Work out the finished part from the listing and answer in its coordinate system (mm). A direction names the side the tool comes from. Coordinates: 2 decimals unless noted, no trailing zeros. Order: outer loops, then holes, each group sorted by start corner. A loop starts at its lowest first (then second) coordinate and runs counter-clockwise, first axis right, second up. Notation, with made-up numbers: (46.5, 71) -> (58.5, 71) arc R26 ccw to (58.5, 99) -> close; hole circle Ø9 at (78.25, 2.5). An arc over 180 degrees is marked (long way). Answer as CSV lines item,"result". Start each with the question number.
Item 1: For a pull along Y with two mould halves and no side action, classify faces 4 (the face through (283, 139.7, 19)), 5 (the face through (343.184, 71.525, 19.317)), 6 (the face through (571.5, 70, 19)) as pulls with the +Y half, pulls with the -Y half, needs draft (parallel to the pull), parting line crosses it, or undercut.
Item 2: Straight lines are drawn through the part: L1, parallel to X at y = 72, z = 19; L2, parallel to Z at x = 527, y = 76; L3, parallel to Y at x = 366, z = 22. For each, find the intervals that lie inside material, in ascending order.
Item 3: Section D-D (y = 99.5) is taken. Write down the section's boundary in (x, z).
Item 4: Section B-B (z = 19.05) is taken. Write down the section's boundary in (x, y).
Item 5: Section C-C (x = 44.45) is taken. Write down the section's boundary in (y, z), then the cut area to 3 significant figures.
Item 6: Section A-A (y = 69.85) is taken. Count the separate pieces of the cut face and the enclosed holes in it, then the cut area to 3 significant figures.
Item 7: Which of the six approach directions +Z, -Z, +X, -X, +Y, -Y give full straight-line access (tool end or side, diameter ignored) to faces 1 (the face through (44, 50.8, 28)), 2 (the face through (526, 50.8, 28)), 3 (the face through (88.9, 114, 19))?
Item 8: Each of these flat-tipped pins is pushed along its axis until it touches: pin 1 Ø19 at (y, z) = (125, 27.5) entering from +X; pin 2 Ø19 at (x, z) = (54.5, 19.5) entering from +Y; pin 3 Ø2 at (y, z) = (122, 4) entering from -X; pin 4 Ø1.5 at (y, z) = (76, 14) entering from -X. Where does it stop, or does it pass through?
```python
from build123d import *

# Parameters (mm, degrees)
SKETCH2_W           = 571.5
SKETCH2_H           = 139.7
BOSS_EXTRUDE2_DEPTH = 38.1
SKETCH3_W           = 88.9
SKETCH3_H           = 50.8
CUT_EXTRUDE1_DEPTH  = 590.559114933
SKETCH4_R           = 38.1
CUT_EXTRUDE2_DEPTH  = 590.559114933
SKETCH5_R           = 4.7625
CUT_EXTRUDE3_DEPTH  = 580.626664328
SKETCH6_R           = 4.7625
CUT_EXTRUDE4_DEPTH  = 580.626664328


with BuildPart() as part:
    # Sketch2 → Boss-Extrude2 (new body)
    with BuildSketch(Plane.XY):
        with Locations((285.75, 69.85)):
            Rectangle(SKETCH2_W, SKETCH2_H)
    extrude(amount=BOSS_EXTRUDE2_DEPTH)

    # Sketch3 → Cut-Extrude1 (cut, through all)
    with BuildSketch(Plane.XY.offset(38.1)):
        with Locations((44.45, 114.3)):
            Rectangle(SKETCH3_W, SKETCH3_H)
        with Locations((527.05, 114.3)):
            Rectangle(SKETCH3_W, SKETCH3_H)
        with Locations((527.05, 25.4)):
            Rectangle(SKETCH3_W, SKETCH3_H)
        with Locations((44.45, 25.4)):
            Rectangle(SKETCH3_W, SKETCH3_H)
    extrude(amount=-CUT_EXTRUDE1_DEPTH, mode=Mode.SUBTRACT)

    # Sketch4 → Cut-Extrude2 (cut, through all)
    with BuildSketch(Plane.XY.offset(38.1)):
        with Locations((381.247583626, 69.85)):
            Circle(SKETCH4_R)
    extrude(amount=-CUT_EXTRUDE2_DEPTH, mode=Mode.SUBTRACT)

    # Sketch5 → Cut-Extrude3 (cut, through all)
    with BuildSketch(Plane(origin=(0, 50.8, 0), x_dir=(-1, 0, 0), z_dir=(0, -1, 0))):
        with Locations(Location((-44.45, -19.05, 0), (0, 0, 180))):
            Circle(SKETCH5_R)
    extrude(amount=-CUT_EXTRUDE3_DEPTH, mode=Mode.SUBTRACT)

    # Sketch6 → Cut-Extrude4 (cut, through all)
    with BuildSketch(Plane.XZ.offset(-50.8)):
        with Locations((527.05, 19.05)):
            Circle(SKETCH6_R)
    extrude(amount=-CUT_EXTRUDE4_DEPTH, mode=Mode.SUBTRACT)


solid = part.part
```
Checked values:
1,face 4,"pulls with the +Y half"
1,face 5,"undercut"
1,face 6,"needs draft"
2,L1,"x = 0 to 39.69, 49.21 to 343.21, 419.29 to 522.29, 531.81 to 571.5"
2,L2,"z = 0 to 14.29, 23.81 to 38.1"
2,L3,"y = 0 to 34.93, 104.77 to 139.7"
3,outline,"(88.9, 0) -> (357.32, 0) -> (357.32, 38.1) -> (88.9, 38.1) -> close; (405.17, 0) -> (482.6, 0) -> (482.6, 38.1) -> (405.17, 38.1) -> close"
4,outline,"(0, 50.8) -> (39.69, 50.8) -> (39.69, 88.9) -> (0, 88.9) -> close; (49.21, 50.8) -> (88.9, 50.8) -> (88.9, 0) -> (482.6, 0) -> (482.6, 50.8) -> (522.29, 50.8) -> (522.29, 88.9) -> (482.6, 88.9) -> (482.6, 139.7) -> (88.9, 139.7) -> (88.9, 88.9) -> (49.21, 88.9) -> close; (531.81, 50.8) -> (571.5, 50.8) -> (571.5, 88.9) -> (531.81, 88.9) -> close; hole circle Ø76.2 at (381.25, 69.85)"
5,outline,"(50.8, 0) -> (88.9, 0) -> (88.9, 14.29) -> (50.8, 14.29) -> close; (50.8, 23.81) -> (88.9, 23.81) -> (88.9, 38.1) -> (50.8, 38.1) -> close"
5,area,"1,090 mm^2"
6,separate pieces,"2"
6,enclosed holes,"2"
6,area,"18,700 mm^2"
7,face 1,"+Z, -Z, -X, -Y"
7,face 2,"+Z, -Z, +X, -Y"
7,face 3,"+Z, -Z, -X, +Y"
8,pin 1,"stops at x = 482.6"
8,pin 2,"stops at y = 88.9"
8,pin 3,"stops at x = 88.9"
8,pin 4,"stops at x = 0"
